Source: CAD feature listing. Evaluate the final solid. Frame: model axes, mm. Face numbers are marked on the shaded views. Give positions to 0.01 mm unless a question says otherwise; leave off trailing zeros. Order: outer loops, then holes, each group sorted by start corner. A loop starts at its lowest first (then second) coordinate and runs counter-clockwise, first axis right, second up. Notation, with made-up numbers: M 4,15.5 L 36,15.5 A31 cw 36,51.5 Z; hole C 60,20.5 d8. An arc over 180 degrees is marked long. Answer in a Markdown table with one row per item. Add a question column.
(1) Section query B-B, the plane x = -10. Return loops of the section in (y, z).
(2) Section query D-D, the plane z = 0. Return loops of the section in (x, y), plus the area to 3 significant figures.
(3) Mould query, pull axis Z, two halves, no side actions, for the marked faces 1, 2, 3 and 4. Classes: pulls with the +Z half, pulls with the -Z half, needs draft (parallel to the pull), parting line crosses it, or undercut.
(4) Section query A-A, the plane z = -1.2. Return loops of the section in (x, y), plus the area to 3 significant figures.
(5) Material intervals for line 1 along X through (y, z) = (4.75, 0); line 2 along X through (y, z) = (3, 0); line 3 along Y through (x, z) = (0, 1.4), sorted ascending.
(6) Section query C-C, the plane y = 6.5. Return loops of the section in (x, z).
(7) Pin query (flat end, axial travel): P1, Ø2, axis at x = -2.5, z = 2, coming from the -Y side; P2, Ø1.8, axis at x = -10, z = 0, coming from the +Y side. Return the tip coordinate at first contact, or that it passes through.
from build123d import *

# Parameters (mm, degrees)
BOSS_EXTRUDE1_DEPTH = 2.6
SKETCH2_R           = 1.5
CUT_EXTRUDE1_DEPTH  = 18.607171834


with BuildPart() as part:
    # Sketch1 → Boss-Extrude1 (new, symmetric)
    with BuildSketch(Plane.XY):
        with BuildLine():
            Line((8, 0), (13.25, 0))
            Line((13.25, 0), (13.25, 11.3))
            Line((13.25, 11.3), (-13.25, 11.3))
            Line((-13.25, 11.3), (-13.25, 0))
            Line((-13.25, 0), (-8, 0))
            ThreePointArc((-8, 0), (0, 8), (8, 0))
        make_face()
    extrude(amount=BOSS_EXTRUDE1_DEPTH, both=True)

    # Sketch2 → Cut-Extrude1 (cut, through all)
    with BuildSketch(Plane(origin=(0, 11.3, 0), x_dir=(1, 0, 0), z_dir=(0, 1, 0))):
        with Locations(Location((-10, 0, 0), (0, 0, 270))):
            Circle(SKETCH2_R)
        with Locations(Location((10, 0, 0), (0, 0, 270))):
            Circle(SKETCH2_R)
    extrude(amount=-CUT_EXTRUDE1_DEPTH, mode=Mode.SUBTRACT)


solid = part.part
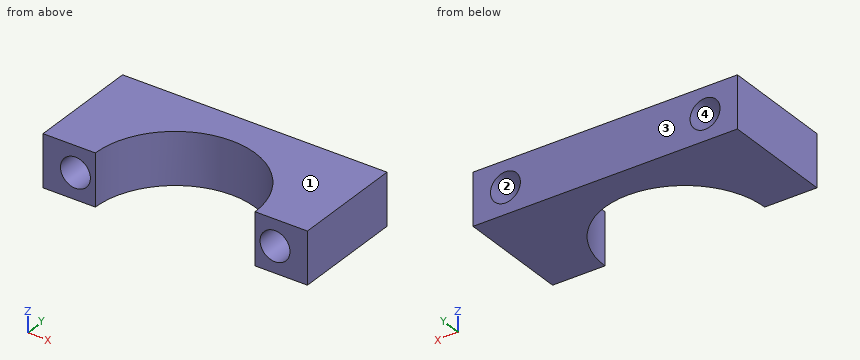
Values follow:
| question | item | result |
|---|---|---|
| 1 | outline | M 0,-2.6 L 11.3,-2.6 L 11.3,-1.5 L 0,-1.5 Z; M 0,1.5 L 11.3,1.5 L 11.3,2.6 L 0,2.6 Z |
| 2 | outline | M -13.25,0 L -11.5,0 L -11.5,11.3 L -13.25,11.3 Z; M -8.5,0 L -8,0 A8 cw 8,0 L 8.5,0 L 8.5,11.3 L -8.5,11.3 Z; M 11.5,0 L 13.25,0 L 13.25,11.3 L 11.5,11.3 Z |
| 2 | area | 131 mm² |
| 3 | face 1 | pulls with the +Z half |
| 3 | face 2 | undercut |
| 3 | face 3 | needs draft |
| 3 | face 4 | undercut |
| 4 | outline | M -13.25,0 L -10.9,0 L -10.9,11.3 L -13.25,11.3 Z; M -9.1,0 L -8,0 A8 cw 8,0 L 9.1,0 L 9.1,11.3 L -9.1,11.3 Z; M 10.9,0 L 13.25,0 L 13.25,11.3 L 10.9,11.3 Z |
| 4 | area | 158 mm² |
| 5 | line 1 | x = -13.25 to -11.5, -8.5 to -6.44, 6.44 to 8.5, 11.5 to 13.25 |
| 5 | line 2 | x = -13.25 to -11.5, -8.5 to -7.42, 7.42 to 8.5, 11.5 to 13.25 |
| 5 | line 3 | y = 8 to 11.3 |
| 6 | outline | M -13.25,-2.6 L -4.66,-2.6 L -4.66,2.6 L -13.25,2.6 Z; M 4.66,-2.6 L 13.25,-2.6 L 13.25,2.6 L 4.66,2.6 Z; hole C -10,0 d3; hole C 10,0 d3 |
| 7 | P1 | stops at y = 7.19 |
| 7 | P2 | passes through |
